Verification items for the finished model (mm, model axes). Face numbers are marked on the shaded views. A direction names the side the tool comes from. Coordinates: 2 decimals unless noted, no trailing zeros. Write each loop counter-clockwise with the first axis right and the second up, starting at its lowest first coordinate (ties: lowest second). Pieces come first, ordered by that corner, then holes. Notation, with made-up numbers: (-26, 43) -> (8, 43) arc R8 ccw to (8, 49) -> close; hole circle Ø5 at (54.5, 17.5). An arc over 180 degrees is marked (long way). Write each question's results on one line, items separated by ' | '. Start each with the question number.
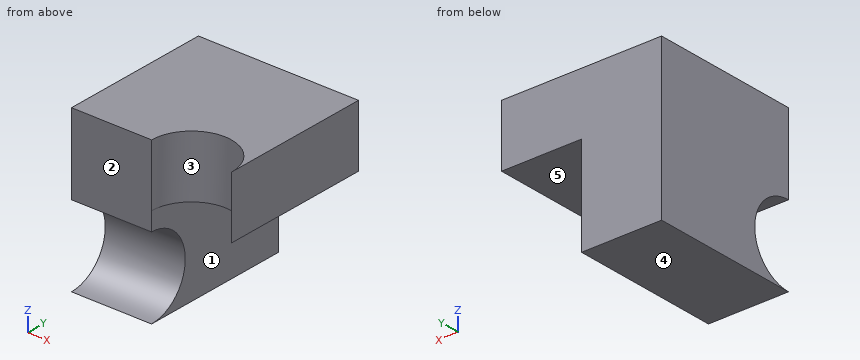
from build123d import *

# Parameters (mm, degrees)
SKETCH1_W               = 25
SKETCH1_H               = 19.246899001
BOSS_EXTRUDE1_DEPTH     = 47
CUT_EXTRUDE1_DEPTH      = 74.034238546
CUT_EXTRUDE1_DEPTH_BACK = 50
SKETCH3_R               = 12.5
CUT_EXTRUDE2_DEPTH      = 50


with BuildPart() as part:
    # Sketch1 → Boss-Extrude1 (new body)
    with BuildSketch(Plane(origin=(0, 0, 0), x_dir=(1, 0, 0), z_dir=(0, 1, 0))):
        Polygon((0, -19.246899001), (0, 0), (0, 30.753100999), (-25, 30.753100999), (-25, -19.246899001), align=None)
        with Locations((12.5, -9.623449501)):
            Rectangle(SKETCH1_W, SKETCH1_H)
    extrude(amount=BOSS_EXTRUDE1_DEPTH)

    # Sketch2 → Cut-Extrude1 (cut, two sides: drawn at the far end of the back side and taken through both)
    with BuildSketch(Plane.XY.offset(19.246899001).offset(-CUT_EXTRUDE1_DEPTH_BACK)):
        with BuildLine():
            Line((25, -147.244307714), (25, 0))
            ThreePointArc((25, 0), (12.5, 12.5), (0, 0))
            Line((0, 0), (0, -147.244307714))
            Line((0, -147.244307714), (0, -441.732923143))
            Line((0, -441.732923143), (25, -441.732923143))
            Line((25, -441.732923143), (25, -147.244307714))
        make_face()
    extrude(amount=CUT_EXTRUDE1_DEPTH + CUT_EXTRUDE1_DEPTH_BACK, mode=Mode.SUBTRACT)

    # Sketch3 → Cut-Extrude2 (cut)
    with BuildSketch(Plane.ZY.offset(25)):
        with Locations((-18.253100999, 0)):
            Circle(SKETCH3_R)
    extrude(amount=-CUT_EXTRUDE2_DEPTH, mode=Mode.SUBTRACT)


solid = part.part
1. Tool access check on the marked faces 4 and 5. Record the directions out of +Z, -Z, +X, -X, +Y, -Y that give a thin tool (end or side, any length) a straight path to the whole face; none if there is none.
2. Mould release check, pull along X, two halves, no side actions. Record for the marked faces 1, 2 and 3: +X half, -X half, draft (parallel to the pull), parting line (faces both ways), or undercut.
3. Sectioned sample at D-D on z = 15.5. Record the cut outline in (x, y).
4. Depth check by flat-ended pin: pin 1 Ø1.5 at (y, z) = (36.5, -24.5) entering from +X; pin 2 Ø20 at (x, y) = (11.5, 18) entering from -Z. Enter the tip coordinate at first touch or a pass-through.
5. Sectioned sample at C-C on y = 9. Record the cut outline in (x, z), plus the area to 3 significant figures.
6. Sectioned sample at A-A on y = 30. Record the cut outline in (x, z), plus the area to 3 significant figures.
7. Sectioned sample at B-B on x = -13. Record the cut outline in (y, z).
8. Material ranges on probe 1 along X at (y, z) = (20, -9); probe 2 along Z at (x, y) = (-14, 2); probe 3 along Z at (x, y) = (-3.5, 7.5), recorded low to high. Write a range as from..to.
Computed values:
1) face 4: -Z, +X, -X, +Y, -Y | face 5: -Z, +X, +Y, -Y
2) face 1: +X half | face 2: draft | face 3: undercut
3) outline: (-25, 0) -> (0, 0) arc R12.5 cw to (25, 0) -> (25, 47) -> (-25, 47) -> close
4) pin 1: stops at x = 0 | pin 2: stops at z = 0
5) outline: (-25, -30.75) -> (0, -30.75) -> (0, -26.93) -> (-25, -26.93) -> close; (-25, -9.58) -> (0, -9.58) -> (0, 0) -> (3.83, 0) -> (3.83, 19.25) -> (-25, 19.25) -> close; (21.17, 0) -> (25, 0) -> (25, 19.25) -> (21.17, 19.25) -> close | area: 964 mm^2
6) outline: (-25, -30.75) -> (0, -30.75) -> (0, 0) -> (25, 0) -> (25, 19.25) -> (-25, 19.25) -> close | area: 1,730 mm^2
7) outline: (0, -30.75) -> (47, -30.75) -> (47, 19.25) -> (0, 19.25) -> (0, -5.75) arc R12.5 cw to start
8) probe 1: x = -25..0 | probe 2: z = -30.75..-30.59, -5.91..19.25 | probe 3: z = -30.75..-28.25, -8.25..19.25
